Can you work these out from the drawing? Everything is in mm from the part's minimum corner. A direction names the side the tool comes from. Round coordinates to 2 decimals unless told otherwise and drop trailing zeros. Loops run counter-clockwise (first coordinate to the right, second up) from the corner with the lowest first, then second, coordinate; pieces in that order, holes last. Notation, with made-up numbers: M 74,-34.75 L 89,-34.75 A30 cw 89,-8.75 Z; hole C -8.75,47 d8. An arc over 180 degrees is marked long. Answer in a Markdown table with one row per item.
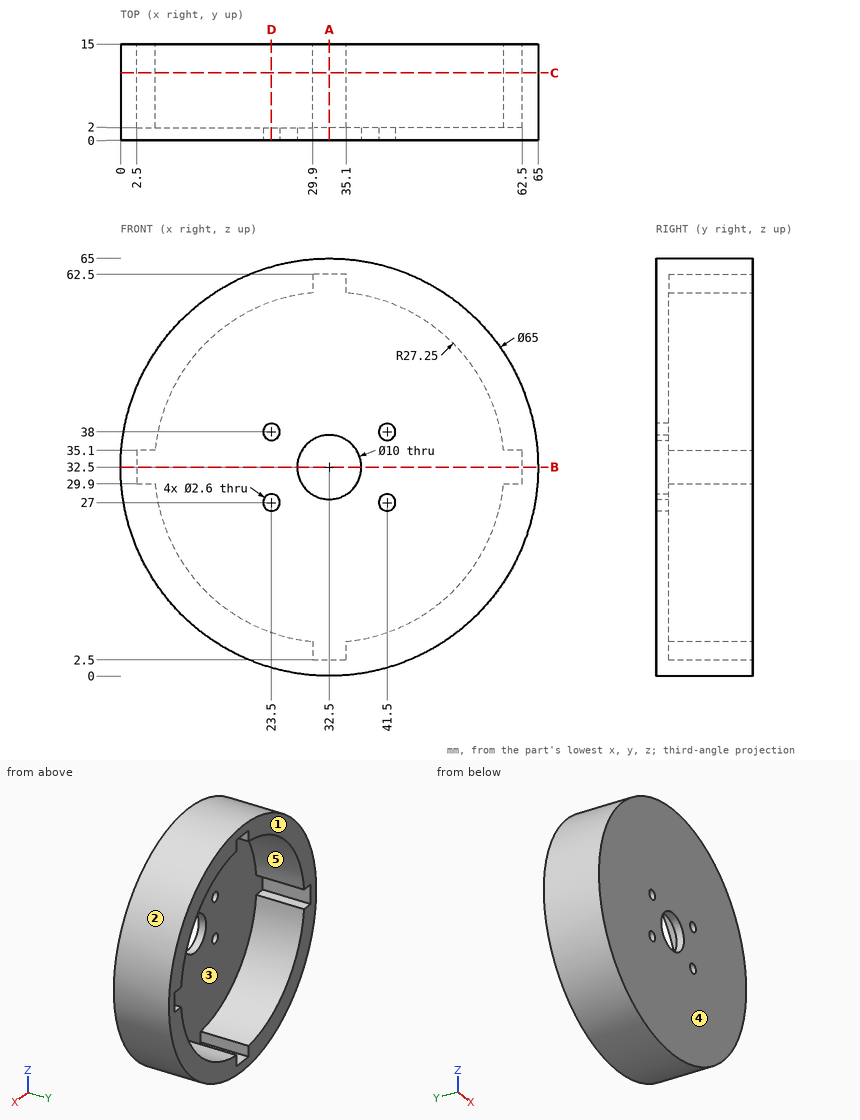
1) I need wall thicknesses on line 1 (X direction, y = 1.6, z = 38); line 2 (X direction, y = 11, z = 32); line 3 (Y direction, x = 28.5, z = 52.5). Which ranges of each line are inside material? Lowest first, please.
Computed:
| item | result |
|---|---|
| line 1 | x = 0.47 to 22.2, 24.8 to 40.2, 42.8 to 64.53 |
| line 2 | x = 0 to 2.5, 62.5 to 65 |
| line 3 | y = 0 to 2 |
2) Will these pins go through, and if not, where does the flat tip stop? P1, Ø2.5, axis at x = 3.5, y = 7.5, coming from the -Z side; P2, Ø3, axis at x = 17.5, y = 9.5, coming from the -Z side; P3, Ø8, axis at y = 4, z = 40.5, coming from the -X side; P4, Ø2.5, axis at x = 33, y = 7.5, coming from the -Z side.
Computed:
| item | result |
|---|---|
| P1 | stops at z = 15.58 |
| P2 | stops at z = 2.94 |
| P3 | stops at x = 0.25 |
| P4 | stops at z = 0 |
3) If we mould it in two halves opening along X, with no side actions, what happens to the marked faces 1, 2 and 3? For each: released by +X, released by -X, zero draft, split by the parting line, or undercut.
Computed:
| item | result |
|---|---|
| face 1 | zero draft |
| face 2 | split by the parting line |
| face 3 | undercut |
4) I want a section at A-A, the plane x = 32.5. Please give me the cut outline in (y, z).
Computed:
| item | result |
|---|---|
| outline | M 0,0 L 15,0 L 15,2.5 L 2,2.5 L 2,27.5 L 0,27.5 Z; M 0,37.5 L 2,37.5 L 2,62.5 L 15,62.5 L 15,65 L 0,65 Z |
5) Which directions (+Z, -Z, +X, -X, +Y, -Y) give clear straight access to the entire face, cutting with the end or side of a thin tool? Please do the marked faces 4 and 5.
Computed:
| item | result |
|---|---|
| face 4 | +Z, -Z, +X, -X, -Y |
| face 5 | +Y |
6) I want a section at C-C, the plane y = 10.5. Please give me the cut outline in (x, z).
Computed:
| item | result |
|---|---|
| outline | C 32.5,32.5 d65; hole M 2.5,29.9 L 5.37,29.9 A27.25 ccw 29.9,5.37 L 29.9,2.5 L 35.1,2.5 L 35.1,5.37 A27.25 ccw 59.63,29.9 L 62.5,29.9 L 62.5,35.1 L 59.63,35.1 A27.25 ccw 35.1,59.63 L 35.1,62.5 L 29.9,62.5 L 29.9,59.63 A27.25 ccw 5.37,35.1 L 2.5,35.1 Z |
7) I want a section at B-B, the plane z = 32.5. Please give me the cut outline in (x, y).
Computed:
| item | result |
|---|---|
| outline | M 0,0 L 27.5,0 L 27.5,2 L 2.5,2 L 2.5,15 L 0,15 Z; M 37.5,0 L 65,0 L 65,15 L 62.5,15 L 62.5,2 L 37.5,2 Z |
8) I want a section at D-D, the plane x = 23.5. Please give me the cut outline in (y, z).
Computed:
| item | result |
|---|---|
| outline | M 0,1.27 L 15,1.27 L 15,6.78 L 2,6.78 L 2,25.7 L 0,25.7 Z; M 0,28.3 L 2,28.3 L 2,36.7 L 0,36.7 Z; M 0,39.3 L 2,39.3 L 2,58.22 L 15,58.22 L 15,63.73 L 0,63.73 Z |
